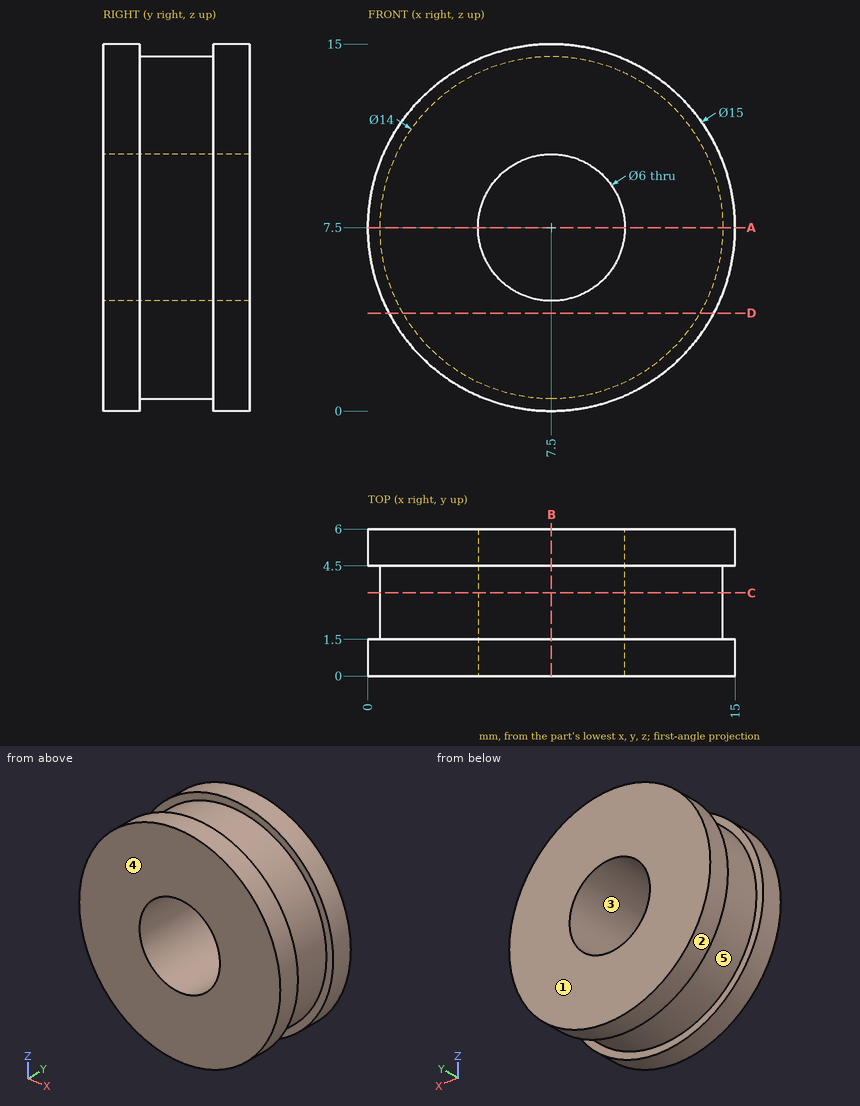
Study the drawing (mm; zero at the part's minimum x, y, z) and answer. A direction names the side the tool comes from. Give positions to 0.01 mm unless a question says otherwise; leave off trailing zeros. Write each loop counter-clockwise with the first axis right and the second up, starting at its lowest first coordinate (ties: lowest second). Pieces come first, ordered by that corner, then holes. Notation, with made-up numbers: (33.25, -1.75) - (48.25, -1.75) arc R28 ccw to (48.25, 20.25) - close; hole circle Ø1 at (50.5, 43.25). An arc over 180 degrees is marked (long way). Write item = value, one per line. Start each with the question number.
Item 1: Find section D-D (z = 4). Give the vertices of the cut face in (x, y).
Item 2: Find section A-A (z = 7.5). Give the vertices of the cut face in (x, y), then the cut area to 3 significant figures.
Item 3: Find section B-B (x = 7.5). Give the vertices of the cut face in (y, z), then the cut area to 3 significant figures.
Item 4: This flat-tipped pin is pushed along its axis until it touches: P1, Ø3, axis at x = 11.5, y = 1.5, coming from the +Z side. Where does it stop, or does it pass through?
Item 5: Find section C-C (y = 3.4). Give the vertices of the cut face in (x, z).
Item 6: A tool of negligible diameter and unlimited length cuts with its end or side. For the marked faces 4 and 5, from which of +Z, -Z, +X, -X, +Y, -Y can it reach the whole face along a straight path? Write none if from no direction.
Item 7: Find the intervals of material crossed by probe 1 along Z at (x, y) = (7.5, 1.3); probe 2 along Z at (x, y) = (9.75, 1.7); probe 3 along X at (y, z) = (3.6, 7.25), in increasing order. Write a range as [from, to].
Item 8: The mould has two halves that part along X. Classify the marked faces 1, 2 and 3: +X half, -X half, draft (parallel to the pull), parting line (faces both ways), or undercut.
Response:
q1.outline = (0.87, 0) - (14.13, 0) - (14.13, 1.5) - (13.56, 1.5) - (13.56, 4.5) - (14.13, 4.5) - (14.13, 6) - (0.87, 6) - (0.87, 4.5) - (1.44, 4.5) - (1.44, 1.5) - (0.87, 1.5) - close
q2.outline = (0, 0) - (4.5, 0) - (4.5, 6) - (0, 6) - (0, 4.5) - (0.5, 4.5) - (0.5, 1.5) - (0, 1.5) - close; (10.5, 0) - (15, 0) - (15, 1.5) - (14.5, 1.5) - (14.5, 4.5) - (15, 4.5) - (15, 6) - (10.5, 6) - close
q2.area = 51.0 mm²
q3.outline = (0, 0) - (1.5, 0) - (1.5, 0.5) - (4.5, 0.5) - (4.5, 0) - (6, 0) - (6, 4.5) - (0, 4.5) - close; (0, 10.5) - (6, 10.5) - (6, 15) - (4.5, 15) - (4.5, 14.5) - (1.5, 14.5) - (1.5, 15) - (0, 15) - close
q3.area = 51.0 mm²
q4.P1 = 14.57
q5.outline = circle Ø14 at (7.5, 7.5); hole circle Ø6 at (7.5, 7.5)
q6.face_4 = +Z, -Z, +X, -X, -Y
q6.face_5 = none
q7.probe_1 = [0, 4.5], [10.5, 15]
q7.probe_2 = [0.87, 5.52], [9.48, 14.13]
q7.probe_3 = [0.5, 4.51], [10.49, 14.5]
q8.face_1 = draft
q8.face_2 = parting line
q8.face_3 = undercut
